Model file for the job. Use its own axes, mm. Face numbers are marked on the shaded views. A direction names the side the tool comes from. Coordinates: 2 decimals unless noted, no trailing zeros. Write each loop counter-clockwise with the first axis right and the second up, starting at its lowest first coordinate (ties: lowest second). Pieces come first, ordered by that corner, then holes. Notation, with made-up numbers: (82.5, 67) -> (107.5, 67) arc R10 cw to (107.5, 71) -> close; hole circle Ø1 at (13.25, 42.5). An arc over 180 degrees is marked (long way). Answer as a JSON object with one key per item and string values. Group by question number.
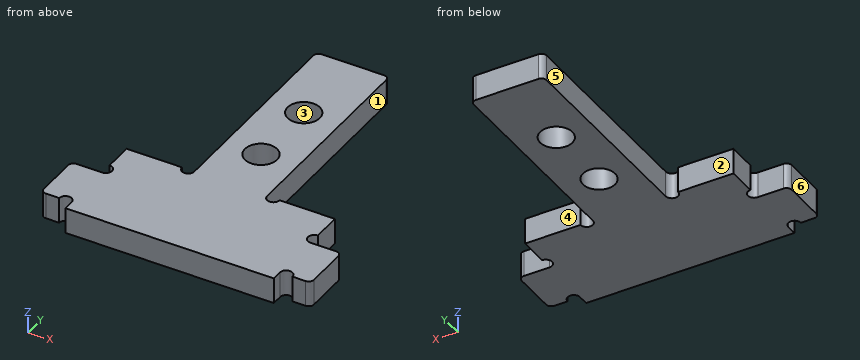
from build123d import *

# Parameters (mm, degrees)
EXTRUDE_1_DEPTH     = 1.25
SKETCH_2_R          = 0.6
CUT_EXTRUDE_1_DEPTH = 3.5
FILLET_1_R          = 0.5
SKETCH_3_R          = 1.55
CUT_EXTRUDE_2_DEPTH = 3.5


with BuildPart() as part:
    # 草图1 → 凸台-拉伸1 (new body, symmetric)
    with BuildSketch(Plane.XY):
        Polygon((-10.025, 6), (-13, 6), (-13, 1), (-10.025, 1), (-10.025, 0), (10.025, 0), (10.025, 1), (13, 1), (13, 6), (10.025, 6), (10.025, 10), (3.5, 10), (3.5, 30), (-3.5, 30), (-3.5, 10), (-10.025, 10), align=None)
    extrude(amount=EXTRUDE_1_DEPTH, both=True)

    # 草图2 → 切除-拉伸1 (cut, through all)
    with BuildSketch(Plane.XY.offset(1.25)):
        with Locations((-10.025, 6.6)):
            Circle(SKETCH_2_R)
        with Locations((-10.625, 1)):
            Circle(SKETCH_2_R)
        with Locations((10.025, 6.6)):
            Circle(SKETCH_2_R)
        with Locations((10.625, 1)):
            Circle(SKETCH_2_R)
        with Locations((-4.1, 10)):
            Circle(SKETCH_2_R)
        with Locations((4.1, 10)):
            Circle(SKETCH_2_R)
    extrude(amount=-CUT_EXTRUDE_1_DEPTH, mode=Mode.SUBTRACT)

    # 圆角1
    fillet_1_edges = [part.edges().sort_by_distance(p)[0] for p in [
        (-3.5, 30, 0),
        (3.5, 30, 0),
        (13, 6, 0),
        (13, 1, 0),
        (-13, 1, 0),
        (-13, 6, 0),
    ]]
    fillet(fillet_1_edges, radius=FILLET_1_R)

    # 草图3 → 切除-拉伸2 (cut, through all)
    with BuildSketch(Plane.XY.offset(1.25)):
        with Locations((0, 14.95)):
            Circle(SKETCH_3_R)
        with Locations((0, 21.95)):
            Circle(SKETCH_3_R)
    extrude(amount=-CUT_EXTRUDE_2_DEPTH, mode=Mode.SUBTRACT)


solid = part.part
(1) Cut at C-C on z = -0.9. Give the number of separate pieces and of enclosed holes in the cut face, plus the area to 3 significant figures.
(2) Pull direction X, two halves, no side cores. Call the marked faces 1, 2 and 3: released by +X, released by -X, zero draft, split by the parting line, or undercut.
(3) Wall check: probe 1 along Y at (x, z) = (0, 0.2); probe 2 along Y at (x, z) = (-1, 1); probe 3 along Y at (x, z) = (-8.5, 0.15). Give the ranges that are in metal, low to high.
(4) Cut at B-B on x = 0. List the corners of the cut face in (y, z).
(5) Cut at A-A on y = 21.95. List the corners of the cut face in (x, z).
(6) Pin check, flat tips, straight feed: pin 1 (1.5 mm diameter, centred on y = 16, z = 0, fed in from +X); pin 2 (1 mm diameter, centred on x = 12, z = 0, fed in from -Y); pin 3 (0.8 mm diameter, centred on y = 8, z = 0, fed in from -X) (3 decimals). Stop position of each tip, or through.
(7) Cut at D-D on x = -4.1. List the corners of the cut face in (y, z), plus the area to 3 significant figures.
(8) 3-axis set-ups, long thin cutter, end or side, ignore diameter. For the marked faces 4, 5 and 6: which of +Z, -Z, +X, -X, +Y, -Y reach the whole face in a straight line?
Results found:
{
 "1": {"separate pieces": "1", "enclosed holes": "2", "area": "351 mm²"},
 "2": {"face 1": "released by +X", "face 2": "zero draft", "face 3": "undercut"},
 "3": {"probe 1": "y = 0 to 13.4, 16.5 to 20.4, 23.5 to 30", "probe 2": "y = 0 to 13.77, 16.13 to 20.77, 23.13 to 30", "probe 3": "y = 0 to 10"},
 "4": {"outline": "(0, -1.25) -> (13.4, -1.25) -> (13.4, 1.25) -> (0, 1.25) -> close; (16.5, -1.25) -> (20.4, -1.25) -> (20.4, 1.25) -> (16.5, 1.25) -> close; (23.5, -1.25) -> (30, -1.25) -> (30, 1.25) -> (23.5, 1.25) -> close"},
 "5": {"outline": "(-3.5, -1.25) -> (-1.55, -1.25) -> (-1.55, 1.25) -> (-3.5, 1.25) -> close; (1.55, -1.25) -> (3.5, -1.25) -> (3.5, 1.25) -> (1.55, 1.25) -> close"},
 "6": {"pin 1": "stops at x = 3.5", "pin 2": "stops at y = 1", "pin 3": "stops at x = -10.025"},
 "7": {"outline": "(0, -1.25) -> (9.4, -1.25) -> (9.4, 1.25) -> (0, 1.25) -> close", "area": "23.5 mm²"},
 "8": {"face 4": "+Z, -Z, +X, +Y", "face 5": "+Z, -Z, -X, +Y", "face 6": "+Z, -Z, -X, +Y, -Y"}
}
